```python
from build123d import *

# Parameters (mm, degrees)
SKETCH_W     = 50
SKETCH_H     = 20
PAD_DEPTH    = 5
SKETCH001_R  = 1.5
HOLE_DEPTH   = 25
SKETCH002_W  = 35
SKETCH002_H  = 10
PAD001_DEPTH = 25
SKETCH003_W  = 27
SKETCH003_H  = 4
POCKET_DEPTH = 11


with BuildPart() as part:
    # Sketch → Pad (new body)
    with BuildSketch(Plane.XY):
        with Locations((0.229687, 0.070392)):
            Rectangle(SKETCH_W, SKETCH_H)
    extrude(amount=PAD_DEPTH)

    # Sketch001 (on Face6 of Pad) → Hole (cut)
    with BuildSketch(Plane.XY.offset(5)):
        with Locations((-21.502412, 0)):
            Circle(SKETCH001_R)
        with Locations((21.629828, 0)):
            Circle(SKETCH001_R)
    extrude(amount=-HOLE_DEPTH, mode=Mode.SUBTRACT)

    # Sketch002 (on Face5 of Hole) → Pad001 (join)
    with BuildSketch(Plane.XY.offset(5)):
        with Locations((-0.013338, 0.040416)):
            Rectangle(SKETCH002_W, SKETCH002_H)
    extrude(amount=PAD001_DEPTH)

    # Sketch003 (on Face12 of Pad001) → Pocket (cut)
    with BuildSketch(Plane(origin=(0, 5.040416, 0), x_dir=(-1, 0, 0), z_dir=(0, 1, 0))):
        with Locations((0.049137, 23.104307)):
            Rectangle(SKETCH003_W, SKETCH003_H)
    extrude(amount=-POCKET_DEPTH, mode=Mode.SUBTRACT)


with BuildPart() as part_1:
    # Body placement: moved
    add(part.part.moved(Location((0, 3, 0))))


solid = part_1.part
```
The listing builds one solid part. Answer for the finished solid, in the listing's coordinates (mm). A direction names the side the tool comes from. Coordinates: 2 decimals unless noted, no trailing zeros. Order: outer loops, then holes, each group sorted by start corner. A loop starts at its lowest first (then second) coordinate and runs counter-clockwise, first axis right, second up. Notation, with made-up numbers: M 15,-11.75 L 59,-11.75 A12 ccw 59,-3.75 Z; hole C 38.25,30 d11. An arc over 180 degrees is marked long. Answer as a JSON object with one key per item and string values. Group by question number.
1. Section C-C on y = -0.5 is taken. Write down the section's boundary in (x, z).
2. Straight lines are drawn through the part: line 1 (Z direction, x = 12, y = 1); line 2 (X direction, y = -1.75, z = 26.25); line 3 (Z direction, x = 5, y = -4). For each, find the intervals that lie inside material, in ascending order.
3. Flat-ended cylindrical pins translate along their axes: P1, Ø4.5, axis at y = 2, z = 22.5, coming from the -X side; P2, Ø5, axis at y = 1, z = 19.5, coming from the +X side; P3, Ø7.5, axis at x = 2, z = 21.5, coming from the -Y side. Find the tip coordinate at first contact, or state that the pin passes through.
4. Section D-D on z = 15 is taken. Write down the section's boundary in (x, y), then the cut area to 3 significant figures.
5. Section A-A on y = 3 is taken. Write down the section's boundary in (x, z).
6. Determine the mould class of faces 1 (the flat face through (17.487, 3, 17)), 2 (the flat face through (0, -1.96, 17)), 3 (the cylindrical face through (-23, 3.1, 2.5)) for opening direction X: released by +X, released by -X, zero draft, split by the parting line, or undercut.
7. Section B-B on x = -4 is taken. Write down the section's boundary in (y, z), then the cut area to 3 significant figures.
8. A tool of negligible diameter and unlimited length cuts with its end or side. For faces 4 (the flat face through (-13.549, 3, 23)), 5 (the flat face through (-17.513, 3, 17)), 6 (the flat face through (0, 8.04, 17)), from which of +Z, -Z, +X, -X, +Y, -Y can it reach the whole face along a straight path? Write none if from no direction.
Values follow:
{
 "1": {"outline": "M -24.77,0 L 25.23,0 L 25.23,5 L 17.49,5 L 17.49,30 L -17.51,30 L -17.51,5 L -24.77,5 Z; hole M -13.55,21.1 L 13.45,21.1 L 13.45,25.1 L -13.55,25.1 Z"},
 "2": {"line 1": "0 to 21.1, 25.1 to 30", "line 2": "-17.51 to 17.49", "line 3": "0 to 5"},
 "3": {"P1": "x = -17.51", "P2": "x = 17.49", "P3": "y = -1.96"},
 "4": {"outline": "M -17.51,-1.96 L 17.49,-1.96 L 17.49,8.04 L -17.51,8.04 Z", "area": "350 mm2"},
 "5": {"outline": "M -24.77,0 L -23,0 L -23,5 L -24.77,5 Z; M -20,0 L 20.13,0 L 20.13,5 L 17.49,5 L 17.49,30 L -17.51,30 L -17.51,5 L -20,5 Z; M 23.13,0 L 25.23,0 L 25.23,5 L 23.13,5 Z; hole M -13.55,21.1 L 13.45,21.1 L 13.45,25.1 L -13.55,25.1 Z"},
 "6": {"face 1": "released by +X", "face 2": "zero draft", "face 3": "undercut"},
 "7": {"outline": "M -6.93,0 L 13.07,0 L 13.07,5 L 8.04,5 L 8.04,21.1 L -1.96,21.1 L -1.96,5 L -6.93,5 Z; M -1.96,25.1 L 8.04,25.1 L 8.04,30 L -1.96,30 Z", "area": "310 mm2"},
 "8": {"face 4": "+Y, -Y", "face 5": "+Z, -X, +Y, -Y", "face 6": "+Z, +X, -X, +Y"}
}
